Autodesk Inventor part; units mm, degrees
ref_plane "YZ Plane" through (0, 0, 0) normal (1, 0, 0) x (0, 1, 0)
ref_plane "XZ Plane" through (0, 0, 0) normal (0, 1, 0) x (-1, 0, 0)
ref_plane "XY Plane" through (0, 0, 0) normal (0, 0, 1) x (1, 0, 0)
sketch "草圖1" plane through (0, 0, 0) normal (0, 0, 1) x (1, 0, 0)
  circle A0 centre (0, 0) radius 60 construction
  circle A1 centre (0, 0) radius 48 construction
  line L0 (350, -100) -> (-100, -100)
  line L1 (-100, -100) -> (-100, 100)
  line L2 (-100, 100) -> (350, 100)
  line L3 (350, 100) -> (350, -100)
  circle A2 centre (0, 54) radius 2.5
  circle A3 centre (-46.7654, 27) radius 2.5
  circle A4 centre (-46.7654, -27) radius 2.5
  circle A5 centre (0, -54) radius 2.5
  circle A6 centre (46.7654, -27) radius 2.5
  circle A7 centre (46.7654, 27) radius 2.5
  circle A8 centre (218.12, -44.54) radius 1.6
  circle A9 centre (136.84, -92.8) radius 1.6
  arc A10 (147.6, -24) -> (143.6, -24) centre (145.6, -24) ccw
  arc A11 (191.4, -24) -> (187.4, -24) centre (189.4, -24) ccw
  arc A12 (143.6, 86) -> (147.6, 86) centre (145.6, 86) ccw
  arc A13 (187.4, 86) -> (191.4, 86) centre (189.4, 86) ccw
  arc A14 (231.2, 86) -> (235.2, 86) centre (233.2, 86) ccw
  arc A15 (235.2, -24) -> (231.2, -24) centre (233.2, -24) ccw
  circle A16 centre (344.5, -27.5) radius 1.75
  arc A17 (257.75, 95) -> (261.25, 95) centre (259.5, 95) ccw
  circle A18 centre (259.5, 95) radius 1.5
  circle A19 centre (233.2, 86) radius 1.5
  circle A20 centre (189.4, 86) radius 1.5
  circle A21 centre (145.6, 86) radius 1.5
  circle A22 centre (145.6, -24) radius 1.5
  circle A23 centre (189.4, -24) radius 1.5
  circle A24 centre (233.2, -24) radius 1.5
  circle A25 centre (218.12, -44.54) radius 1.5
  circle A26 centre (136.84, -92.8) radius 1.5
  circle A27 centre (344.5, -27.5) radius 1.5
  circle A28 centre (0, -54) radius 3.275
  circle A29 centre (0, 54) radius 3.275
  circle A30 centre (46.7654, -27) radius 3.275
  circle A31 centre (-46.7654, -27) radius 3.275
  circle A32 centre (-46.7654, 27) radius 3.275
  circle A33 centre (46.7654, 27) radius 3.275
  point P0 (0, 0)
  dimension "d0" = 450
  dimension "d1" = 200
  dimension "d2" = 100
  dimension "d3" = 100
  dimension "d6" = 5
  dimension "d9" = 360
  dimension "d14" = 3
  dimension "d15" = 3
  dimension "d16" = 3
  dimension "d17" = 3
  dimension "d18" = 3
  dimension "d19" = 3
  dimension "d20" = 3
  dimension "d21" = 3
  dimension "d22" = 3
  dimension "d23" = 3
extrude "擠出1" add sketch "草圖1" along normal blind 6 contours L0 L1 L2 L3 | A28 | A29 | A30 | A31 | A32 | A33
chamfer "倒角1" distance 2.5 angle 45 6 edges at (-2.5, -54, 6) (-49.2654, -27, 6) (-49.2654, 27, 6) (-2.5, 54, 6) (44.2654, 27, 6) (44.2654, -27, 6)
sketch "草圖2" plane through (0, 0, 0) normal (0, 0, -1) x (-1, 0, 0)
  line L0 (-350, 100) -> (100, 100)
  line L1 (-350, -100) -> (-350, 100)
  line L2 (100, -100) -> (-350, -100)
  line L3 (100, 100) -> (100, -100)
  circle A0 centre (0, 54) radius 2.5
  circle A1 centre (46.7654, 27) radius 2.5
  circle A2 centre (46.7654, -27) radius 2.5
  circle A3 centre (0, -54) radius 2.5
  circle A4 centre (-46.7654, -27) radius 2.5
  circle A5 centre (-46.7654, 27) radius 2.5
  circle A6 centre (-233.2, -24) radius 1.5
  circle A7 centre (-189.4, -24) radius 1.5
  circle A8 centre (-145.6, -24) radius 1.5
  circle A9 centre (-145.6, 86) radius 1.5
  circle A10 centre (-189.4, 86) radius 1.5
  circle A11 centre (-233.2, 86) radius 1.5
  circle A12 centre (-259.5, 95) radius 1.5
  circle A13 centre (-344.5, -27.5) radius 1.75
  circle A14 centre (-136.84, -92.8) radius 1.6
  circle A15 centre (-218.12, -44.54) radius 1.6
  point P0 (0, 0)
properties part number "base plate"
The listing builds one solid part. Answer for the finished solid, in the listing's coordinates (mm). Give positions to 0.01 mm unless a question says otherwise; leave off trailing zeros. Use one line per item in the form item = value. Start each with the question number.
(1) Consider line 1 (X direction, y = 86, z = 3.2); line 2 (Y direction, x = -46.5, z = 4.2); line 3 (X direction, y = -43.5, z = 1.55). Determine where each line is inside the solid, lowest interval first. Write a range as from..to.
(2) The mould has two halves that part along Y. Classify faces 1 (the flat face through (122, 1, 0)), 2 (the conical face through (-47.341, 24.407, 3.656)): released by +Y, released by -Y, zero draft, split by the parting line, or undercut.
(3) Flat-ended cylindrical pins translate along their axes: pin 1 Ø4.5 at (x, y) = (0, -54) entering from -Z; pin 2 Ø6 at (x, y) = (46.77, -27) entering from +Z. Find the tip coordinate at first contact, or state that the pin passes through.
Ans:
q1.line_1 = -100..144.1, 147.1..187.9, 190.9..231.7, 234.7..350
q1.line_2 = -100..-30.19, -23.81..23.81, 30.19..100
q1.line_3 = -100..216.9, 219.34..350
q2.face_1 = zero draft
q2.face_2 = undercut
q3.pin_1 = through
q3.pin_2 = 4
